from build123d import *

# Parameters (mm, degrees)
SKETCH1_R               = 7.9375
BOSS_EXTRUDE1_DEPTH     = 6.35
SKETCH2_R               = 6.6675
BOSS_EXTRUDE2_DEPTH     = 12.7
CUT_EXTRUDE1_DEPTH      = 23.11131639
CUT_EXTRUDE1_DEPTH_BACK = 23.11131639
SKETCH5_R               = 3.4544


with BuildPart() as part:
    # Sketch1 → Boss-Extrude1 (new body)
    with BuildSketch(Plane(origin=(0, 0, 0), x_dir=(1, 0, 0), z_dir=(0, 1, 0))):
        with Locations(Location((0, 0, 0), (0, 0, 270))):
            Circle(SKETCH1_R)
    extrude(amount=BOSS_EXTRUDE1_DEPTH)

    # Sketch2 → Boss-Extrude2 (add)
    with BuildSketch(Plane.XZ):
        with Locations(Location((0, 0, 0), (0, 0, 270))):
            Circle(SKETCH2_R)
    extrude(amount=BOSS_EXTRUDE2_DEPTH)

    # Sketch5 → Cut-Extrude1 (cut, two sides: drawn at the far end of the back side and taken through both)
    with BuildSketch(Plane(origin=(0, 6.35, 0), x_dir=(1, 0, 0), z_dir=(0, 1, 0)).offset(-CUT_EXTRUDE1_DEPTH_BACK)):
        with Locations(Location((0, 0, 0), (0, 0, 270))):
            Circle(SKETCH5_R)
    extrude(amount=CUT_EXTRUDE1_DEPTH + CUT_EXTRUDE1_DEPTH_BACK, mode=Mode.SUBTRACT)


solid = part.part
Could you check a few things on this model? Use its own coordinates, in mm. A direction names the side the tool comes from. Coordinates: 2 decimals unless noted, no trailing zeros. Order: outer loops, then holes, each group sorted by start corner. A loop starts at its lowest first (then second) coordinate and runs counter-clockwise, first axis right, second up. Notation, with made-up numbers: (38, 43.25) -> (94, 43.25) arc R32 cw to (94, 72.25) -> close; hole circle Ø5 at (42, 84). An arc over 180 degrees is marked (long way). One line per item, written item: value. Start each with the question number.
1) Which directions (+Z, -Z, +X, -X, +Y, -Y) give clear straight access to the entire face, cutting with the end or side of a thin tool? Please do faces 1 (the flat face through (-2, 6.35, 3)), 2 (the flat face through (7, 0, -2)).
2) Imagine slicing it at B-B on z = 0. List the corners of the cut face in (x, y) for me, plus the area to 3 significant figures.
3) Imagine slicing it at C-C on y = -3.5. List the corners of the cut face in (x, z) for me (1 decimal).
4) If I drill on L1, parallel to X at y = -4.5, z = 0; L2, parallel to Z at x = -0.25, y = -6; L3, parallel to X at y = 2, z = -1.25, over which ranges is the centre line in solid material (lowest first)? Write a range as [from, to].
5) I'm going to push flat-ended pins straight in: pin 1 (1.5 mm diameter, centred on x = 5.5, y = -4.5, fed in from -Z); pin 2 (1.5 mm diameter, centred on x = -6.5, z = -4, fed in from -Y); pin 3 (5 mm diameter, centred on y = 3, z = -3.5, fed in from -X). Where does each tip first touch, or does it pass through?
6) Imagine slicing it at D-D on x = 5.75. List the corners of the cut face in (y, z) for me, plus the area to 3 significant figures.
7) Imagine slicing it at A-A on x = 0. List the corners of the cut face in (y, z) for me.
Answer list:
1. face 1: +Z, -Z, +X, -X, +Y
1. face 2: -Y
2. outline: (-7.94, 0) -> (-6.67, 0) -> (-6.67, -12.7) -> (-3.45, -12.7) -> (-3.45, 6.35) -> (-7.94, 6.35) -> close; (3.45, -12.7) -> (6.67, -12.7) -> (6.67, 0) -> (7.94, 0) -> (7.94, 6.35) -> (3.45, 6.35) -> close
2. area: 139 mm2
3. outline: circle Ø13.3 at (0, 0); hole circle Ø6.9 at (0, 0)
4. L1: x = [-6.67, -3.45], [3.45, 6.67]
4. L2: z = [-6.66, -3.45], [3.45, 6.66]
4. L3: x = [-7.84, -3.22], [3.22, 7.84]
5. pin 1: stops at z = -4.68
5. pin 2: stops at y = 0
5. pin 3: stops at x = -7.87
6. outline: (-12.7, -3.38) -> (0, -3.38) -> (0, -5.47) -> (6.35, -5.47) -> (6.35, 5.47) -> (0, 5.47) -> (0, 3.38) -> (-12.7, 3.38) -> close
6. area: 155 mm2
7. outline: (-12.7, -6.67) -> (0, -6.67) -> (0, -7.94) -> (6.35, -7.94) -> (6.35, -3.45) -> (-12.7, -3.45) -> close; (-12.7, 3.45) -> (6.35, 3.45) -> (6.35, 7.94) -> (0, 7.94) -> (0, 6.67) -> (-12.7, 6.67) -> close
